from build123d import *

# Parameters (mm, degrees)
F0_W       = 1
F0_H       = 1
F0_W_2     = 20
F0_H_2     = 3
F0_W_3     = 3
F0_H_3     = 10
F1_DEPTH   = 25
F2_SIZE2   = 0.49999
F2_SIZE    = 0.99999
F2_2_SIZE2 = 0.5
F2_2_SIZE  = 1
F3_SIZE2   = 1
F3_SIZE    = 0.5
F3_2_SIZE2 = 0.99999
F3_2_SIZE  = 0.49999


# Not quite as in the source:
# - a fillet or chamfer is up to 0.001 mm smaller than in the source, because OpenCascade refuses the exact size


with BuildPart() as f1:
    # F0 (on Top) → F1 (new body)
    with BuildSketch(Plane.XY):
        Polygon((-12.6065595312, 12.1843403429), (-15.6065595312, 12.1843403429), (-15.6065595312, -10.8156596571), (-12.6065595312, -10.8156596571), (-12.6065595312, -7.8156596571), (-12.6065595312, 11.1843403429), align=None)
        with Locations((-12.1065595312, 11.6843403429)):
            Rectangle(F0_W, F0_H)
        with Locations((-2.6065595312, -9.3156596571)):
            Rectangle(F0_W_2, F0_H_2)
        Polygon((7.3934404688, -7.8156596571), (7.3934404688, -10.8156596571), (10.3934404688, -10.8156596571), (10.3934404688, 12.1843403429), (7.3934404688, 12.1843403429), (7.3934404688, 11.1843403429), align=None)
        with Locations((-14.1065595312, -15.8156596571)):
            Rectangle(F0_W_3, F0_H_3)
        Polygon((-12.6065595312, -20.8156596571), (-15.6065595312, -20.8156596571), (-15.6065595312, -23.8156596571), (10.3934404688, -23.8156596571), (10.3934404688, -20.8156596571), align=None)
        with Locations((6.8934404688, 11.6843403429)):
            Rectangle(F0_W, F0_H)
    extrude(amount=F1_DEPTH)

    # F2 (size 1 and 0.5 in the source; OpenCascade refuses exactly that, so slightly less here)
    f2_edges = [f1.edges().sort_by_distance(p)[0] for p in [
        (6.39344, 11.18434, 12.5),
    ]]
    f2_side = f1.faces().sort_by_distance((6.89344, 11.18434, 12.5))[0]
    chamfer(f2_edges, length=F2_SIZE, length2=F2_SIZE2, reference=f2_side)

    # F2#2
    f2_2_edges = [f1.edges().sort_by_distance(p)[0] for p in [
        (-11.60656, 12.18434, 12.5),
    ]]
    f2_2_side = f1.faces().sort_by_distance((-13.60656, 12.18434, 12.5))[0]
    chamfer(f2_2_edges, length=F2_2_SIZE, length2=F2_2_SIZE2, reference=f2_2_side)

    # F3
    f3_edges = [f1.edges().sort_by_distance(p)[0] for p in [
        (6.39344, 12.18434, 12.5),
    ]]
    f3_side = f1.faces().sort_by_distance((6.39344, 11.934335, 12.5))[0]
    chamfer(f3_edges, length=F3_SIZE, length2=F3_SIZE2, reference=f3_side)

    # F3#2 (size 0.5 and 1 in the source; OpenCascade refuses exactly that, so slightly less here)
    f3_2_edges = [f1.edges().sort_by_distance(p)[0] for p in [
        (-11.60656, 11.18434, 12.5),
    ]]
    f3_2_side = f1.faces().sort_by_distance((-11.60656, 11.43434, 12.5))[0]
    chamfer(f3_2_edges, length=F3_2_SIZE, length2=F3_2_SIZE2, reference=f3_2_side)


solid = f1.part
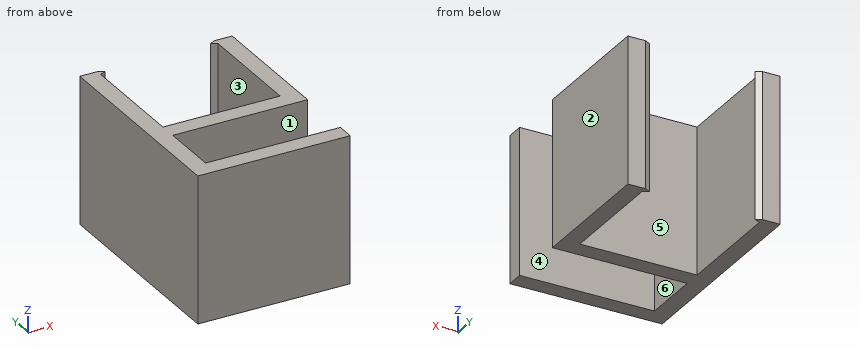
Input: part model. Units: mm. Frame: model coordinates. Face numbers are marked on the shaded views. A direction names the side the tool comes from. Give positions to 0.01 mm unless a question says otherwise; leave off trailing zeros. Order: outer loops, then holes, each group sorted by start corner. A loop starts at its lowest first (then second) coordinate and runs counter-clockwise, first axis right, second up. Notation, with made-up numbers: (58, 36) - (95, 36) arc R16 ccw to (95, 41) - close; hole circle Ø10 at (-32, 32.5). An arc over 180 degrees is marked (long way). Answer as a JSON object with one key per item and string values. Group by question number.
Q1. Cut plane B-B, the plane x = 3.5. Output: boundary loops of the cut face in (y, z).
Q2. Mould query, pull axis X, two halves, no side actions, for the marked faces 4, 5 and 6. Classes: pulls with the +X half, pulls with the -X half, needs draft (parallel to the pull), parting line crosses it, or undercut.
Q3. Line query: probe 1 along Y at (x, z) = (6.25, 21.25); probe 2 along X at (y, z) = (9.5, 18); probe 3 along Y at (x, z) = (-12.25, 1.75). Output: solid intervals per line, ascending.
Q4. First-contact query: pin 1 Ø10 at (x, z) = (2, 6.5) entering from +Y; pin 2 Ø11 at (y, z) = (-15.5, 10) entering from +X; pin 3 Ø5 at (x, z) = (-3, 15.5) entering from +Y. Flat tips, straight axial feed; report the tip coordinate or a pass-through.
Q5. Cut plane D-D, the plane y = -17. Output: boundary loops of the cut face in (x, z).
Q6. Set-up query: the marked faces 1, 2 and 3. Return all of +Z, -Z, +X, -X, +Y, -Y with unobstructed straight access to the full face (end or side cutting, diameter ignored); none if empty.
Q7. Cut plane A-A, the plane y = 0. Output: boundary loops of the cut face in (x, z).
Results:
{
 "1": {"outline": "(-23.82, 0) - (-20.82, 0) - (-20.82, 25) - (-23.82, 25) - close; (-10.82, 0) - (-7.82, 0) - (-7.82, 25) - (-10.82, 25) - close"},
 "2": {"face 4": "needs draft", "face 5": "undercut", "face 6": "pulls with the +X half"},
 "3": {"probe 1": "-23.82 to -20.82, -10.82 to -7.82", "probe 2": "-15.61 to -12.61, 7.39 to 10.39", "probe 3": "-23.82 to -20.82, -10.82 to -7.82, 11.36 to 12.01"},
 "4": {"pin 1": "y = 11.99", "pin 2": "x = 10.39", "pin 3": "y = -7.82"},
 "5": {"outline": "(-15.61, 0) - (-12.61, 0) - (-12.61, 25) - (-15.61, 25) - close"},
 "6": {"face 1": "+Z, -Z, +X", "face 2": "+Z, -Z, +X, +Y, -Y", "face 3": "+Z, -Z"},
 "7": {"outline": "(-15.61, 0) - (-12.61, 0) - (-12.61, 25) - (-15.61, 25) - close; (7.39, 0) - (10.39, 0) - (10.39, 25) - (7.39, 25) - close"}
}
